Check sheet for the modelled part. Datum: model origin and axes. Units: mm. Give positions to 0.01 mm unless a question says otherwise; leave off trailing zeros. Loops run counter-clockwise (first coordinate to the right, second up) from the corner with the lowest first, then second, coordinate; pieces in that order, holes last. Notation, with made-up numbers: (-25, 33) - (32, 33) arc R19 cw to (32, 60) - close; hole circle Ø3 at (-6, 54). An arc over 180 degrees is marked (long way). Use one line per item in the form item = value.
from build123d import *

# Parameters (mm, degrees)
BOSS_EXTRUDE1_DEPTH = 24
FILLET1_R           = 3.5


with BuildPart() as part:
    # Sketch2 → Boss-Extrude1 (new body)
    with BuildSketch(Plane(origin=(0, 0, 0), x_dir=(1, 0, 0), z_dir=(0, 1, 0))):
        with BuildLine():
            ThreePointArc((11.591585182, 1.269721351), (-3.263225558, -10.020142683), (-19.529660289, -0.880693402))
            Line((-19.529660289, -0.880693402), (-19.773089177, -1.006807758))
            Line((-19.773089177, -1.006807758), (-22.163972243, -2.245463863))
            ThreePointArc((-22.163972243, -2.245463863), (0.291704356, -12.459871192), (15.531753085, 6.939418571))
            ThreePointArc((15.531753085, 6.939418571), (15.503757233, 7.996392633), (15.419848185, 9.050402694))
            Line((15.419848185, 9.050402694), (12.469626172, 8.736734142))
            ThreePointArc((12.469626172, 8.736734142), (12.517251304, 5.667453249), (12.012150504, 2.639644382))
            ThreePointArc((12.012150504, 2.639644382), (11.918925763, 2.297657269), (11.818590923, 1.957688215))
            ThreePointArc((11.818590923, 1.957688215), (11.708753165, 1.61249542), (11.591585182, 1.269721351))
        make_face()
    extrude(amount=BOSS_EXTRUDE1_DEPTH)

    # Fillet1
    # the kernel refuses this fillet: 3.5 mm, written as the material it takes off along each edge
    with BuildSketch(Plane(origin=(-4.43509674, 0, -6.939418571), x_dir=(-0.9990167342617219, 0, 0.04433468918402287), z_dir=(-0.04433468918402287, 0, -0.9990167342617219))) as fillet1_piece_1:
        with BuildLine():
            CenterArc((16.466849825, 3.45915465), FILLET1_R, 278.761897774, 81.238102226)
            Line((17, 0), (17.010663004, -0.069183093))
            ThreePointArc((17.010663004, -0.069183093), (18.483424912, -0.07), (19.966849825, -0.07))
            Line((19.966849825, -0.07), (20.036849825, 0))
            Line((20.036849825, 0), (20.036849825, 3.45915465))
            Line((20.036849825, 3.45915465), (19.966849825, 3.45915465))
        make_face()
    revolve(axis=Axis((-4.43509674, 0, -6.939418571), (0, 1, 0)), revolution_arc=208.374392147, mode=Mode.SUBTRACT)
    with BuildSketch(Plane(origin=(-4.43509674, 24, -6.939418571), x_dir=(0.85792670476254, 0, -0.5137720985566359), z_dir=(-0.5137720985566359, 0, -0.85792670476254))) as fillet1_piece_2:
        with BuildLine():
            CenterArc((16.466849825, 3.45915465), FILLET1_R, 278.761897774, 81.238102226)
            Line((19.966849825, 3.45915465), (20.036849825, 3.45915465))
            Line((20.036849825, 3.45915465), (20.036849825, 0))
            Line((20.036849825, 0), (19.966849825, -0.07))
            ThreePointArc((19.966849825, -0.07), (18.483424912, -0.07), (17.010663004, -0.069183093))
            Line((17.010663004, -0.069183093), (17, 0))
        make_face()
    revolve(axis=Axis((-4.43509674, 24, -6.939418571), (0, -1, 0)), revolution_arc=208.374392147, mode=Mode.SUBTRACT)


solid = part.part
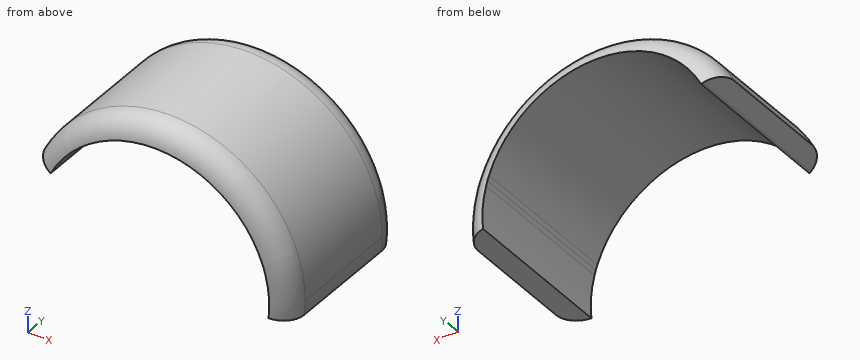
Item 1: Section check B-B on y = 22.5. Record the boundary of the cut face in (x, z), then the cut area to 3 significant figures.
Answer block:
outline = (-21.63, 1.97) - (-19.53, 0.88) arc R17 cw to (11.59, -1.27) arc R17 cw to (11.82, -1.96) arc R17 cw to (12.01, -2.64) arc R17 cw to (12.47, -8.74) - (14.82, -8.99) arc R19.37 ccw to start
area = 119 mm2
Item 2: Thickness scan on L1, parallel to X at y = 9, z = 5.75; L2, parallel to X at y = 9.5, z = 8.5; L3, parallel to Z at x = -4, y = 16.25. Record the ranges inside material, lowest first.
Answer block:
L1 = -19.85 to -15.75, 6.88 to 10.98
L2 = -17.1 to -11.55, 2.68 to 8.23
L3 = 10.06 to 13.02
Item 3: Section check A-A on y = 6. Record the boundary of the cut face in (x, z), then the cut area to 3 significant figures.
Answer block:
outline = (-22.16, 2.25) - (-19.53, 0.88) arc R17 cw to (11.59, -1.27) arc R17 cw to (11.82, -1.96) arc R17 cw to (12.01, -2.64) arc R17 cw to (12.47, -8.74) - (15.42, -9.05) arc R19.97 ccw to start
area = 152 mm2
Item 4: Gauge pin test, flat ends, axial feed: P1, Ø1.5, axis at y = 9, z = 6.5, coming from the -X side; P2, Ø8, axis at x = 1.5, y = 20.5, coming from the -Z side; P3, Ø6, axis at x = -8, y = 21.5, coming from the -Z side. Record the tip position at first contact, or that the pin passes through.
Answer block:
P1 = -19.85
P2 = 6.86
P3 = 8.74
